Print and shaded views of the part. All mm, measured from the part's lowest x, y and z. A direction names the side the tool comes from. Give positions to 0.01 mm unless a question says otherwise; leave off trailing zeros. Write each loop counter-clockwise with the first axis right and the second up, starting at its lowest first coordinate (ties: lowest second). Pieces come first, ordered by that corner, then holes. Notation, with made-up numbers: M 20.25,84.5 L 34.25,84.5 A30 ccw 34.25,113.5 Z; hole C -38,19 d1. An arc over 180 degrees is marked long. One line per question, with ' | ' between items. Start each with the question number.
1. Cut at A-A, the plane z = 8. Write the cut outline in (x, y).
2. Cut at D-D, the plane z = 42. Count the separate pieces of the cut face and the enclosed holes in it, then the cut area to 3 significant figures.
3. Wall check: L1, parallel to X at y = 14, z = 45; L2, parallel to Z at x = 3.25, y = 52; L3, parallel to Y at x = 26.5, z = 45.5. Give the ranges that are in metal, low to high.
4. Cut at C-C, the plane y = 52. Write the cut outline in (x, z).
5. Cut at B-B, the plane x = 42. Write the cut outline in (y, z), then the cut area to 3 significant figures.
6. Flat gauge pins, fed straight in: pin 1 (6 mm diameter, centred on x = 73, z = 45, fed in from +Y); pin 2 (21.5 mm diameter, centred on x = 52, z = 27, fed in from -Y). Where does each tip first touch, or does it go through?
7. Which spindle directions (+Z, -Z, +X, -X, +Y, -Y) get a long thin tool onto all of the face, cutting with end or side? Do the marked faces 1, 2 and 3. Say none if no direction does.
8. Pull direction Z, two halves, no side cores. Call the marked faces 4, 5 and 6: released by +Z, released by -Z, zero draft, split by the parting line, or undercut.
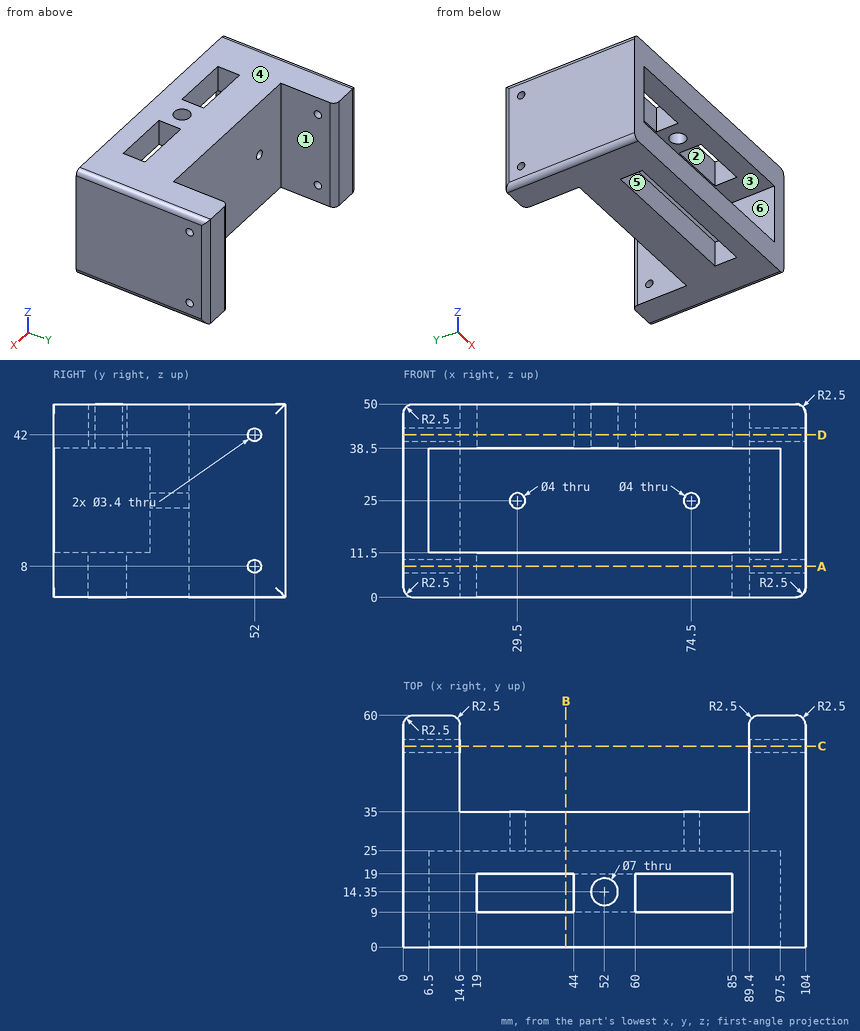
Here are the results:
1) outline: M 0,0 L 104,0 L 104,50.3 L 89.4,50.3 L 89.4,35 L 14.6,35 L 14.6,50.3 L 0,50.3 Z; M 0,53.7 L 14.6,53.7 L 14.6,57.5 A2.5 ccw 12.1,60 L 2.5,60 A2.5 ccw 0,57.5 Z; M 89.4,53.7 L 104,53.7 L 104,57.5 A2.5 ccw 101.5,60 L 91.9,60 A2.5 ccw 89.4,57.5 Z; hole M 19,9 L 85,9 L 85,19 L 19,19 Z
2) separate pieces: 3 | enclosed holes: 3 | area: 3,730 mm^2
3) L1: 0 to 19, 44 to 48.52, 55.48 to 60, 85 to 104 | L2: 0 to 6.3, 9.7 to 40.3, 43.7 to 50 | L3: 0 to 9, 19 to 35
4) outline: M 0,2.5 A2.5 ccw 2.5,0 L 14.6,0 L 14.6,6.3 L 0,6.3 Z; M 0,9.7 L 14.6,9.7 L 14.6,40.3 L 0,40.3 Z; M 0,43.7 L 14.6,43.7 L 14.6,50 L 2.5,50 A2.5 ccw 0,47.5 Z; M 89.4,0 L 101.5,0 A2.5 ccw 104,2.5 L 104,6.3 L 89.4,6.3 Z; M 89.4,9.7 L 104,9.7 L 104,40.3 L 89.4,40.3 Z; M 89.4,43.7 L 104,43.7 L 104,47.5 A2.5 ccw 101.5,50 L 89.4,50 Z
5) outline: M 0,0 L 9,0 L 9,11.5 L 0,11.5 Z; M 0,38.5 L 9,38.5 L 9,50 L 0,50 Z; M 19,0 L 35,0 L 35,50 L 19,50 L 19,38.5 L 25,38.5 L 25,11.5 L 19,11.5 Z | area: 845 mm^2
6) pin 1: y = 35 | pin 2: y = 25
7) face 1: +Z, -Z, +Y | face 2: +Z, -Z | face 3: -Y
8) face 4: released by +Z | face 5: zero draft | face 6: undercut
